Build history of the part. All positions in model axes, mm. Face numbers are marked on the shaded views. Give positions to 0.01 mm unless a question says otherwise; leave off trailing zeros. Loops run counter-clockwise (first coordinate to the right, second up) from the corner with the lowest first, then second, coordinate; pieces in that order, holes last.
1) Band-saw the part on B-B on z = 394.5. List the corners of the cut face in (x, y).
2) Two-plate mould, pull along Y, no slides. Class the marked faces 1, 2 and 3: +Y half, -Y half, draft (parallel to the pull), parting line (faces both ways), or undercut.
3) Wall check: line 1 (X direction, y = 457, z = 366); line 2 (Y direction, x = -2, z = 352); line 3 (Z direction, x = 2, y = 373.5). Give the ranges that are in metal, low to high.
4) Band-saw the part on D-D on x = 41.5. List the corners of the cut face in (y, z), then the cut area to 3 significant figures.
5) Flat gauge pins, fed straight in: P1, Ø1.5, axis at x = -26, y = 223, coming from the -Z side; P2, Ø1, axis at x = 6.5, z = 401, coming from the -Y side; P3, Ø10, axis at x = 26, y = 74.5, coming from the -Z side. Where does each tip first touch, or does it go through?
6) Band-saw the part on C-C on y = 118. List the corners of the cut face in (x, z), then the cut area to 3 significant figures.
7) Band-saw the part on A-A on x = 0. List the corners of the cut face in (y, z), then the cut area to 3 significant figures.
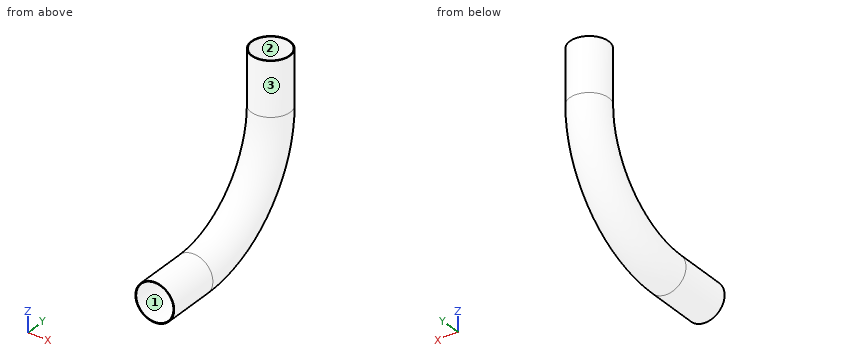
Autodesk Inventor part; units mm, degrees
ref_plane "Work Plane4" through (-55, 152.4, 0) normal (-1, 0, 0) x (0, -1, 0)
ref_plane "YZ Plane" through (0, 0, 0) normal (1, 0, 0) x (0, 1, 0)
ref_plane "XZ Plane" through (0, 0, 0) normal (0, 1, 0) x (-1, 0, 0)
sketch "Sketch1" plane through (0, 0, 0) normal (0, 1, 0) x (-1, 0, 0)
  circle A0 centre (0, 0) radius 55
  circle A1 centre (0, 0) radius 52.7
  dimension "d0" = 110
  dimension "d1" = 2.3
extrude "Extrusion1" add sketch "Sketch1" along normal blind 152.4
sketch "Sketch4" plane through (0, 152.4, 0) normal (0, 1, 0) x (1, 0, 0)
  circle A0 centre (0, 0) radius 52.7
  circle A1 centre (0, 0) radius 55
  point P0 (-55, 0)
ref_plane "Work Plane4" through (-55, 152.4, 0) normal (-1, 0, 0) x (0, -1, 0)
sketch "Sketch8" plane through (-55, 152.4, 0) normal (-1, 0, 0) x (0, -1, 0)
  line L0 (0, 0) -> (0, 304.8) construction
  arc A0 (-304.8, 304.8) -> (0, 0) centre (0, 304.8) ccw
  line L1 (0, 304.8) -> (-304.8, 304.8) construction
  point P0 (152.4, 0)
  dimension "d7" = 304.8
sweep "Sweep1" add profiles "Sketch4" path "Sketch8"
sketch "Sketch9" plane through (0, 457.2, 304.8) normal (0, 0, 1) x (1, 0, 0)
  circle A0 centre (0, 0) radius 52.7
  circle A1 centre (0, 0) radius 55
  point P0 (0, -457.2)
extrude "Extrusion2" add sketch "Sketch9" along normal blind 152.4
properties part number "sweep"
Findings below:
1. outline: circle Ø110 at (0, 457.2); hole circle Ø105.4 at (0, 457.2)
2. face 1: draft
2. face 2: undercut
2. face 3: parting line
3. line 1: x = -55 to -52.7, 52.7 to 55
3. line 2: y = 402.24 to 404.54, 509.86 to 512.16
3. line 3: z = 21 to 23.92, 183.6 to 188.47
4. outline: (0, -36.09) - (152.4, -36.09) arc R340.89 ccw to (493.29, 304.8) - (493.29, 457.2) - (489.68, 457.2) - (489.68, 304.8) arc R337.28 cw to (152.4, -32.48) - (0, -32.48) - close; (0, 32.48) - (152.4, 32.48) arc R272.32 ccw to (424.72, 304.8) - (424.72, 457.2) - (421.11, 457.2) - (421.11, 304.8) arc R268.71 cw to (152.4, 36.09) - (0, 36.09) - close
4. area: 5,660 mm2
5. P1: stops at z = -41.77
5. P2: stops at y = 402.53
5. P3: stops at z = -50.83
6. outline: circle Ø110 at (0, 0); hole circle Ø105.4 at (0, 0)
6. area: 778 mm2
7. outline: (0, -55) - (152.4, -55) arc R359.8 ccw to (512.2, 304.8) - (512.2, 457.2) - (509.9, 457.2) - (509.9, 304.8) arc R357.5 cw to (152.4, -52.7) - (0, -52.7) - close; (0, 52.7) - (152.4, 52.7) arc R252.1 ccw to (404.5, 304.8) - (404.5, 457.2) - (402.2, 457.2) - (402.2, 304.8) arc R249.8 cw to (152.4, 55) - (0, 55) - close
7. area: 3,600 mm2
